```python
from build123d import *

# Parameters (mm, degrees)
SKETCH_W        = 18
SKETCH_H        = 10
PAD_DEPTH       = 13
SKETCH009_R     = 1.5
POCKET_DEPTH    = 4
POCKET001_DEPTH = 2.5
POCKET002_DEPTH = 10.001
SKETCH012_R     = 1.5
POCKET003_DEPTH = 10.001


with BuildPart() as part:
    # Sketch → Pad (new body)
    with BuildSketch(Plane.XY):
        with Locations((9, 5)):
            Rectangle(SKETCH_W, SKETCH_H)
    extrude(amount=PAD_DEPTH)

    # Sketch009 (on DatumPlane) → Pocket (cut, symmetric)
    with BuildSketch(Plane.XY.offset(9)):
        with Locations((3, 5)):
            Circle(SKETCH009_R)
        with Locations((15, 5)):
            Circle(SKETCH009_R)
    extrude(amount=POCKET_DEPTH, both=True, mode=Mode.SUBTRACT)

    # Sketch010 (on DatumPlane) → Pocket001 (cut)
    with BuildSketch(Plane.XY.offset(9)):
        Polygon((4.732051, 2), (6.464102, 5), (4.732051, 8), (1.267949, 8), (0, 8), (0, 2), (1.267949, 2), align=None)
        Polygon((16.732051, 8), (13.267949, 8), (11.535898, 5), (13.267949, 2), (16.732051, 2), (18, 2), (18, 8), align=None)
    extrude(amount=-POCKET001_DEPTH, mode=Mode.SUBTRACT)

    # Sketch011 → Pocket002 (cut, through all)
    with BuildSketch(Plane.XZ):
        Polygon((6.45, 0), (11.55, 0), (13.917136, 4.1), (4.082864, 4.1), align=None)
    extrude(amount=-POCKET002_DEPTH, mode=Mode.SUBTRACT)

    # Sketch012 → Pocket003 (cut, through all)
    with BuildSketch(Plane.XZ):
        with Locations((9, 8.5)):
            Circle(SKETCH012_R)
    extrude(amount=-POCKET003_DEPTH, mode=Mode.SUBTRACT)


solid = part.part
```
Verification items for the finished model (mm, model axes). A direction names the side the tool comes from. Coordinates: 2 decimals unless noted, no trailing zeros. Loops run counter-clockwise (first coordinate to the right, second up) from the corner with the lowest first, then second, coordinate; pieces in that order, holes last. Notation, with made-up numbers: (39.25, 60) -> (83.25, 60) arc R16 ccw to (83.25, 68) -> close; hole circle Ø8 at (-35, 13). An arc over 180 degrees is marked (long way). Answer in a Markdown table with one row per item.
1) Section check A-A (x = 9). Record the cut outline in (y, z), and give its area (3 significant figures).
The answers:
| item | result |
|---|---|
| outline | (0, 4.1) -> (10, 4.1) -> (10, 7) -> (0, 7) -> close; (0, 10) -> (10, 10) -> (10, 13) -> (0, 13) -> close |
| area | 59.0 mm2 |
2) Scan lines: line 1 along Z through (x, y) = (15, 7.75); line 2 along Y through (x, z) = (15, 5.55); line 3 along X through (y, z) = (6, 12.25). Record each from-to range of solid material in increasing order. Write a range as from..to.
The answers:
| item | result |
|---|---|
| line 1 | z = 0..6.5, 9..13 |
| line 2 | y = 0..3.5, 6.5..10 |
| line 3 | x = 0..1.88, 4.12..13.88, 16.12..18 |
3) Section check D-D (x = 17.25). Record the cut outline in (y, z), and give its area (3 significant figures).
The answers:
| item | result |
|---|---|
| outline | (0, 0) -> (10, 0) -> (10, 13) -> (0, 13) -> close; hole (2, 6.5) -> (8, 6.5) -> (8, 9) -> (2, 9) -> close |
| area | 115 mm2 |
4) Section check C-C (y = 2.25). Record the cut outline in (x, z).
The answers:
| item | result |
|---|---|
| outline | (0, 0) -> (6.45, 0) -> (4.08, 4.1) -> (13.92, 4.1) -> (11.55, 0) -> (18, 0) -> (18, 6.5) -> (13.12, 6.5) -> (13.12, 9) -> (18, 9) -> (18, 13) -> (0, 13) -> (0, 9) -> (4.88, 9) -> (4.88, 6.5) -> (0, 6.5) -> close; hole circle Ø3 at (9, 8.5) |
5) Draft check along Z on faces 1 (the face through (3, 5, 0)), 2 (the face through (5.6, 3.5, 7.8)), 3 (the face through (0, 5, 6)). Enter one of: released by +Z, released by -Z, zero draft, split by the parting line, or undercut.
The answers:
| item | result |
|---|---|
| face 1 | released by -Z |
| face 2 | undercut |
| face 3 | zero draft |
6) Depth check by flat-ended pin: P1, Ø1.5, axis at x = 3, y = 5, coming from the +Z side; P2, Ø2, axis at x = 10, y = 2.5, coming from the -Z side. Enter the tip coordinate at first touch or a pass-through.
The answers:
| item | result |
|---|---|
| P1 | stops at z = 5 |
| P2 | stops at z = 4.1 |
7) Access from +Z, -Z, +X, -X, +Y, -Y to the whole of each face (thin tool, end or side, straight path). Record for faces 4 (the face through (5.6, 6.5, 7.8)), 5 (the face through (16.2, 6.4, 6.5)), 6 (the face through (5.25, 4.93, 2.08)), 7 (the face through (13.5, 5.07, 11.03)).
The answers:
| item | result |
|---|---|
| face 4 | -X |
| face 5 | +X |
| face 6 | +Y, -Y |
| face 7 | +Z |
8) Section check B-B (z = 8.5). Record the cut outline in (x, y), and give its area (3 significant figures).
The answers:
| item | result |
|---|---|
| outline | (0, 0) -> (7.5, 0) -> (7.5, 10) -> (0, 10) -> (0, 8) -> (4.73, 8) -> (6.46, 5) -> (4.73, 2) -> (0, 2) -> close; (10.5, 0) -> (18, 0) -> (18, 2) -> (13.27, 2) -> (11.54, 5) -> (13.27, 8) -> (18, 8) -> (18, 10) -> (10.5, 10) -> close |
| area | 82.8 mm2 |
